Answer from the drawing. Dimensions are ordinates in mm from the lowest x, y and z of the part. Round coordinates to 2 decimals unless told otherwise and drop trailing zeros. Write each loop counter-clockwise with the first axis right and the second up, starting at its lowest first coordinate (ties: lowest second). Pieces come first, ordered by that corner, then holes. Notation, with made-up numbers: (-34, 6.5) - (-26, 6.5) arc R30 cw to (-26, 36.5) - close; hole circle Ø8 at (-39.75, 3.5). An arc over 180 degrees is marked (long way). Return JSON: item names as keys, results as strings. Group by question number.
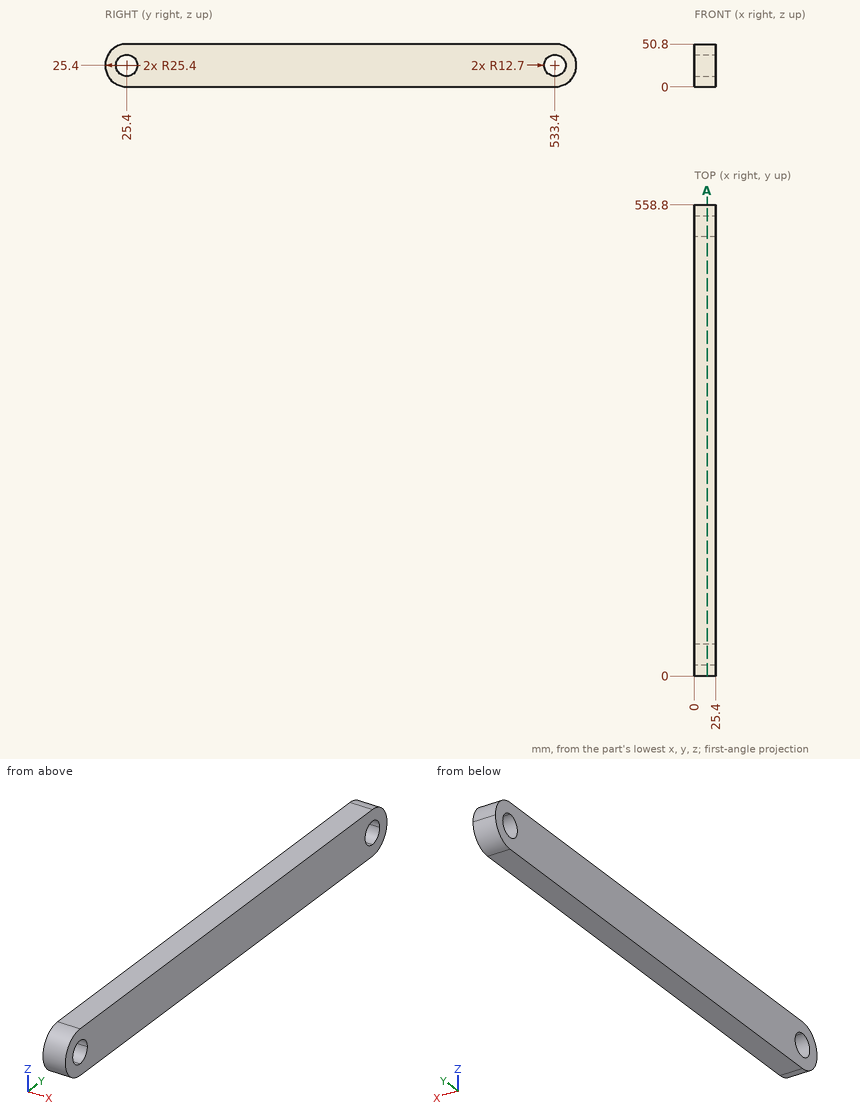
(1) Find section A-A (x = 15.25). Write down the section's boundary in (y, z), plus the area to 3 significant figures.
(2) A flat-ended cylindrical pin translates along its axis: pin 1 (4 mm diameter, centred on x = 12, z = 28, fed in from +Y). Find the tip coordinate at first contact, or state that the pin passes through.
(3) Consider line 1 (Z direction, x = 20, y = 27); line 2 (Y direction, x = 13, z = 14.5); line 3 (Y direction, x = 16.5, z = 32). Determine where each line is inside the solid, lowest interval first.
Check sheet entries:
{
 "1": {"outline": "(25.4, 0) - (533.4, 0) arc R25.4 ccw to (533.4, 50.8) - (25.4, 50.8) arc R25.4 ccw to start; hole circle Ø25.4 at (25.4, 25.4); hole circle Ø25.4 at (533.4, 25.4)", "area": "26,800 mm^2"},
 "2": {"pin 1": "stops at y = 558.79"},
 "3": {"line 1": "z = 0 to 12.8, 38 to 50.8", "line 2": "y = 2.46 to 18.88, 31.92 to 526.88, 539.92 to 556.34", "line 3": "y = 0.87 to 14.55, 36.25 to 522.55, 544.25 to 557.93"}
}
